For this review, take the finished solid that the model builds, in its own axes (mm). Coordinates: 2 decimals unless noted, no trailing zeros. Loops run counter-clockwise (first coordinate to the right, second up) from the corner with the lowest first, then second, coordinate; pieces in that order, holes last. Notation, with made-up numbers: M -6.5,15.25 L 33.5,15.25 A33 ccw 33.5,49.25 Z; hole C 10,2.5 d1. An arc over 180 degrees is marked long. Use one line per item in the form item = value.
Autodesk Inventor part; units mm, degrees
ref_plane "YZ Plane" through (0, 0, 0) normal (1, 0, 0) x (0, 1, 0)
ref_plane "XZ Plane" through (0, 0, 0) normal (0, 1, 0) x (-1, 0, 0)
ref_plane "XY Plane" through (0, 0, 0) normal (0, 0, 1) x (1, 0, 0)
sketch "Szkic1" plane through (0, 0, 0) normal (0, 1, 0) x (-1, 0, 0)
  line L0 (0, 0) -> (0, -75) construction
  line L1 (-56.5, -37.5) -> (56.5, -37.5) construction
  line L2 (56.5, -10) -> (56.5, -65) construction
  line L3 (-56.5, -10) -> (-56.5, -65) construction
  circle A0 centre (56.5, -10) radius 5
  circle A1 centre (56.5, -65) radius 5
  circle A2 centre (0, 0) radius 5
  circle A3 centre (0, -75) radius 5
  circle A4 centre (-56.5, -10) radius 5
  circle A5 centre (-56.5, -65) radius 5
  line L4 (0.8714, 4.9235) -> (57.3714, -5.0765)
  line L5 (57.3714, -69.9235) -> (0.8714, -79.9235)
  line L6 (-0.8714, -79.9235) -> (-57.3714, -69.9235)
  line L7 (-57.3714, -5.0765) -> (-0.8714, 4.9235)
  line L8 (-61.5, -10) -> (-61.5, -65)
  line L9 (61.5, -10) -> (61.5, -65)
  point P0 (0, -37.5)
  point P1 (0, -37.5)
  dimension "d0" = 75
  dimension "d1" = 113
  dimension "d2" = 55
  dimension "d3" = 55
  dimension "d4" = 10
  dimension "d5" = 10
  dimension "d6" = 10
  dimension "d7" = 10
  dimension "d8" = 10
  dimension "d9" = 10
extrude "Wyciągnięcie proste1" add sketch "Szkic1" along normal blind 2
sketch "Szkic2" plane through (0, 2, 0) normal (0, 1, 0) x (1, 0, 0)
  arc A0 (-0.8714, -4.9235) -> (0.8714, -4.9235) centre (0, 0) ccw
  arc A1 (0.8714, 79.9235) -> (-0.8714, 79.9235) centre (0, 75) ccw
  arc A2 (61.5, 65) -> (57.3714, 69.9235) centre (56.5, 65) ccw
  arc A3 (57.3714, 5.0765) -> (61.5, 10) centre (56.5, 10) ccw
  arc A4 (-61.5, 10) -> (-57.3714, 5.0765) centre (-56.5, 10) ccw
  arc A5 (-57.3714, 69.9235) -> (-61.5, 65) centre (-56.5, 65) ccw
hole "Otwór1" at (-56.5, 2, -65) at (-56.5, 2, -10) at (0, 2, 0) at (56.5, 2, -10) at (0, 2, -75) at (56.5, 2, -65) direction (0, -1, 0) diameter 3.5 depth 8
sketch "Szkic3" plane through (0, 2, 0) normal (0, 1, 0) x (1, 0, 0)
  circle A0 centre (0, 75) radius 1.75
  circle A1 centre (0, 0) radius 1.75
  circle A2 centre (-56.5, 65) radius 1.75
  circle A3 centre (-56.5, 10) radius 1.75
  circle A4 centre (56.5, 10) radius 1.75
  circle A5 centre (56.5, 65) radius 1.75
  arc A6 (-61.5, 10) -> (-57.3714, 5.0765) centre (-56.5, 10) ccw
  line L0 (-57.3714, 5.0765) -> (-0.8714, -4.9235)
  arc A7 (-0.8714, -4.9235) -> (0.8714, -4.9235) centre (0, 0) ccw
  line L1 (0.8714, -4.9235) -> (57.3714, 5.0765)
  arc A8 (57.3714, 5.0765) -> (61.5, 10) centre (56.5, 10) ccw
  line L2 (61.5, 10) -> (61.5, 65)
  arc A9 (61.5, 65) -> (57.3714, 69.9235) centre (56.5, 65) ccw
  line L3 (57.3714, 69.9235) -> (0.8714, 79.9235)
  arc A10 (0.8714, 79.9235) -> (-0.8714, 79.9235) centre (0, 75) ccw
  line L4 (-0.8714, 79.9235) -> (-57.3714, 69.9235)
  arc A11 (-57.3714, 69.9235) -> (-61.5, 65) centre (-56.5, 65) ccw
  line L5 (-61.5, 65) -> (-61.5, 10)
  line L6 (0, 5.0777) -> (-51.5, 14.1928)
  line L7 (-51.5, 14.1928) -> (-51.5, 60.8072)
  line L8 (-51.5, 60.8072) -> (0, 69.9223)
  line L9 (0, 69.9223) -> (51.5, 60.8072)
  line L10 (51.5, 60.8072) -> (51.5, 14.1928)
  line L11 (51.5, 14.1928) -> (0, 5.0777)
  circle A12 centre (0, 0) radius 1.75
  circle A13 centre (0, 75) radius 1.75
  line L12 (0, 0) -> (0, 75) construction
  line L13 (4.0221, 0) -> (4.0221, 75)
  line L14 (-4.0221, 75) -> (-4.0221, 0)
  arc A14 (-4.0221, 0) -> (4.0221, 0) centre (0, 0) ccw
  arc A15 (4.0221, 75) -> (-4.0221, 75) centre (0, 75) ccw
  point P0 (0, 37.5)
  point P1 (4.0221, 69.2104)
  point P2 (4.0221, 5.7896)
  point P3 (-4.0221, 5.7896)
  point P4 (-4.0221, 69.2104)
  dimension "d19" = 10
extrude "Wyciągnięcie proste2" cut sketch "Szkic3" against normal through all contours L6 L7 L8 L14 | L13 L9 L10 L11
fillet "Zaokrąglenie1" radius 3 8 edges at (-51.5, 1, -60.8072) (-51.5, 1, -14.1928) (-4.0221, 1, -5.7896) (4.0221, 1, -5.7896) (-4.0221, 1, -69.2104) (4.0221, 1, -69.2104) (51.5, 1, -60.8072) (51.5, 1, -14.1928)
properties part number "podstawa"
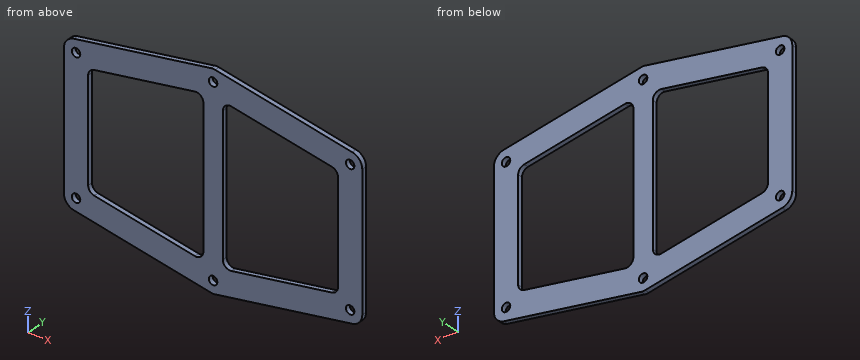
1. Consider section A-A on z = -30. Write out the cut boundary in (x, y).
Computed values:
outline = M -61.5,0 L -51.5,0 L -51.5,2 L -61.5,2 Z; M -4.02,0 L 4.02,0 L 4.02,2 L -4.02,2 Z; M 51.5,0 L 61.5,0 L 61.5,2 L 51.5,2 Z
2. Consider section B-B on x = -23. Write out the cut boundary in (y, z), plus the area to 3 significant figures.
Computed values:
outline = M 0,-76.01 L 2,-76.01 L 2,-65.85 L 0,-65.85 Z; M 0,-9.15 L 2,-9.15 L 2,1.01 L 0,1.01 Z
area = 40.6 mm2
3. Consider section D-D on y = 0.9. State how many separate pieces and enclosed holes the cut face has, plus the area to 3 significant figures.
Computed values:
separate_pieces = 1
enclosed_holes = 8
area = 3,860 mm2
4. Consider section C-C on z = 0. Write out the cut boundary in (x, y), plus the area to 3 significant figures.
Computed values:
outline = M -28.69,0 L -1.75,0 L -1.75,2 L -28.69,2 Z; M 1.75,0 L 28.69,0 L 28.69,2 L 1.75,2 Z
area = 108 mm2
5. Wall thickness on line 1 along X through (y, z) = (0.65, -46); line 2 along Z through (x, y) = (56.5, 1.5); line 3 along X through (y, z) = (1.85, -15): over which ranges is each line inside the solid? List them lowest first. Write a range as from..to.
Computed values:
line_1 = -61.5..-51.5, -4.02..4.02, 51.5..61.5
line_2 = -70.08..-66.75, -63.25..-11.75, -8.25..-4.92
line_3 = -61.5..-50.97, -4.02..4.02, 50.97..61.5
